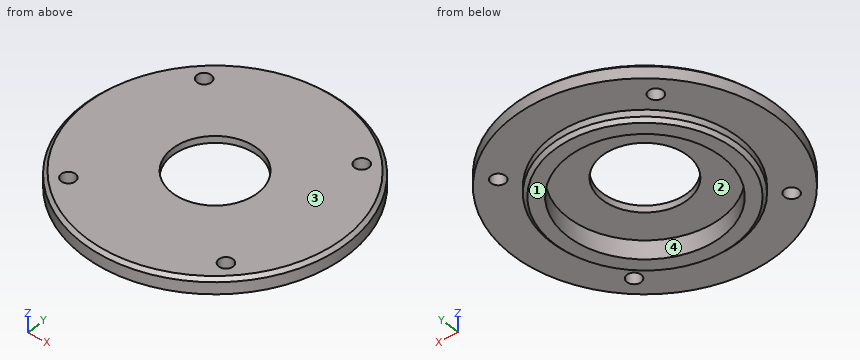
Autodesk Inventor part; units mm, degrees
ref_plane "YZ Plane" through (0, 0, 0) normal (1, 0, 0) x (0, 1, 0)
ref_plane "XZ Plane" through (0, 0, 0) normal (0, 1, 0) x (-1, 0, 0)
ref_plane "XY Plane" through (0, 0, 0) normal (0, 0, 1) x (1, 0, 0)
sketch "Эскиз1" plane through (0, 0, 0) normal (0, 1, 0) x (-1, 0, 0)
  line L0 (0, 0) -> (77.5, 0)
  line L1 (77.5, 0) -> (77.5, -9)
  line L2 (77.5, -9) -> (55, -9)
  line L3 (55, -9) -> (55, -15)
  line L4 (0, -4) -> (0, 0)
  line L5 (55, -15) -> (45, -15)
  line L6 (45, -15) -> (45, -4)
  line L7 (45, -4) -> (0, -4)
  dimension "d0" = 155
  dimension "d1" = 110
  dimension "d3" = 9
  dimension "d5" = 15
  dimension "d6" = 90
  dimension "d7" = 4
revolve "Вращение1" add sketch "Эскиз1" angle 360 about axis through (0, 0, -4) along (0, 0, 1)
sketch "Эскиз3" plane through (0, 0, 0) normal (0, 0, 1) x (1, 0, 0)
  circle A0 centre (0, 0) radius 66.25 construction
  line L0 (0, 0) -> (-70.023, -70.023) construction
  line L1 (0, 0) -> (99.0274, 0) construction
  point P0 (0, 0)
  point P1 (-46.8458, -46.8458)
  point P2 (46.8458, -46.8458)
  point P3 (46.8458, 46.8458)
  point P4 (-46.8458, 46.8458)
  dimension "d15" = 132.5
  dimension "d16" = 135
  dimension "d19" = 360
hole "Отверстие1" at (-46.8458, -46.8458, 0) at (46.8458, -46.8458, 0) at (46.8458, 46.8458, 0) at (-46.8458, 46.8458, 0) direction (0, 0, -1) diameter 8.376 end through all
chamfer "Фаска1" distance 2 angle 45 2 edges at (55, 0, -15) (77.5, 0, 0)
sketch "Эскиз4" plane through (0, 0, 0) normal (0, 0, 1) x (1, 0, 0)
  circle A0 centre (0, 0) radius 77.5
  point P0 (0, 0)
hole "Отверстие2" at (0, 0, 0) direction (0, 0, -1) diameter 50 end through all
properties part number "МПСТ Крышка подшипника с отверстием 110" material "Сталь, углеродистая"
Can you work these out from the model? Positions are in its coordinate system, mm. Face numbers are marked on the shaded views. A direction names the side the tool comes from. Round coordinates to 2 decimals unless told otherwise and drop trailing zeros. Loops run counter-clockwise (first coordinate to the right, second up) from the corner with the lowest first, then second, coordinate; pieces in that order, holes last. Notation, with made-up numbers: M 36,6.5 L 71,6.5 A20 ccw 71,20.5 Z; hole C 85.25,24 d7. An arc over 180 degrees is marked long. Answer as a JSON object with one key per item and string values. Group by question number.
Q1. Imagine slicing it at C-C, the plane z = -6. Please give me the cut outline in (x, y).
Q2. Will these pins go through, and if not, where does the flat tip stop? pin 1 (8 mm diameter, centred on x = 30, z = -12.5, fed in from -Y); pin 2 (4 mm diameter, centred on x = 19.5, y = 36.5, fed in from -Z); pin 3 (11 mm diameter, centred on x = 46.85, y = -46.85, fed in from -Z); pin 4 (1.5 mm diameter, centred on x = 56.5, z = -13, fed in from +Y).
Q3. Imagine slicing it at A-A, the plane x = 0. Please give me the cut outline in (y, z), then the cut area to 3 significant figures.
Q4. We'd pull the mould along Y, two halves only. Please class the marked faces 1 and 2: +Y half, -Y half, draft (parallel to the pull), parting line (faces both ways), or undercut.
Q5. On a 3-axis mill with a long thin cutter (end or side, diameter ignored), from which of +Z, -Z, +X, -X, +Y, -Y can I reach the whole of each face in a straight line? I mean the marked faces 3 and 4. Say none if no direction works.
Q6. Please list where these lines run through material, in increasing order: L1, parallel to Y at x = 0, z = -2.5; L2, parallel to Z at x = 3, y = -64.5.
Findings:
{
 "1": {"outline": "C 0,0 d155; hole C -46.85,-46.85 d8.38; hole C -46.85,46.85 d8.38; hole C 0,0 d90; hole C 46.85,-46.85 d8.38; hole C 46.85,46.85 d8.38"},
 "2": {"pin 1": "stops at y = -72.24", "pin 2": "stops at z = -4", "pin 3": "stops at z = -9", "pin 4": "passes through"},
 "3": {"outline": "M -77.5,-9 L -55,-9 L -55,-13 L -53,-15 L -45,-15 L -45,-4 L -25,-4 L -25,0 L -75.5,0 L -77.5,-2 Z; M 25,-4 L 45,-4 L 45,-15 L 53,-15 L 55,-13 L 55,-9 L 77.5,-9 L 77.5,-2 L 75.5,0 L 25,0 Z", "area": "857 mm2"},
 "4": {"face 1": "draft", "face 2": "undercut"},
 "5": {"face 3": "+Z, +X, -X, +Y, -Y", "face 4": "-Z"},
 "6": {"L1": "y = -77.5 to -25, 25 to 77.5", "L2": "z = -9 to 0"}
}
